```python
from build123d import *

# Parameters (mm, degrees)
EXTRUDE_1_DEPTH      = 30
EXTRUDE_1_DEPTH_BACK = 30
SKETCH_3_R           = 3.15
CUT_EXTRUDE_1_DEPTH  = 89.119294142


with BuildPart() as part:
    # Sketch 1 → Extrude 1 (new, two sides: drawn at the far end of the back side and taken through both)
    with BuildSketch(Plane.XY.offset(-EXTRUDE_1_DEPTH_BACK)):
        Polygon((-37.55, 0), (37.55, 0), (37.55, 35), (32.7, 35), (32.7, 5), (-32.7, 5), (-32.7, 35), (-37.55, 35), align=None)
    extrude(amount=EXTRUDE_1_DEPTH + EXTRUDE_1_DEPTH_BACK)

    # Sketch 3 → Cut-Extrude 1 (cut, through all)
    with BuildSketch(Plane.ZY.offset(37.55)):
        with Locations(Location((10, 27, 0), (0, 0, 270))):
            Circle(SKETCH_3_R)
        with BuildLine():
            Line((30, 5), (17.149177618, 30.590161471))
            ThreePointArc((17.149177618, 30.590161471), (14.199923108, 33.808865242), (10, 35))
            Line((10, 35), (30, 35))
            Line((30, 35), (30, 5))
        make_face()
        with BuildLine():
            ThreePointArc((-2.8, 27), (0.949033201, 17.949033201), (10, 14.2))
            ThreePointArc((10, 14.2), (12.2, 12), (10, 9.8))
            ThreePointArc((10, 9.8), (-2.162236636, 14.837763364), (-7.2, 27))
            ThreePointArc((-7.2, 27), (-5, 29.2), (-2.8, 27))
        make_face()
    extrude(amount=-CUT_EXTRUDE_1_DEPTH, mode=Mode.SUBTRACT)


solid = part.part
```
Work out the finished part from the listing and answer in its coordinate system (mm). A direction names the side the tool comes from. Round coordinates to 2 decimals unless told otherwise and drop trailing zeros. Write each loop counter-clockwise with the first axis right and the second up, starting at its lowest first coordinate (ties: lowest second). Pieces come first, ordered by that corner, then holes.
1) A cutting plane is placed at A-A on y = 21.5. Determine the outline of the cut face in (x, z), and give its area (3 significant figures).
2) Which of the six approach directions +Z, -Z, +X, -X, +Y, -Y give full straight-line access (tool end or side, diameter ignored) to faces 1 (the face through (-35, 35, -10)), 2 (the face through (-35.159, 14.705, -2.028)), 3 (the face through (0, 5, 0))?
3) A cutting plane is placed at B-B on z = -5. Determine the outline of the cut face in (x, y).
4) Determine the mould class of faces 4 (the face through (-32.7, 20, -7)), 5 (the face through (-35.2, 29.2, -5)), 6 (the face through (-1, 0, 0)), 7 (the face through (35.09, 33.78, 14.25)) for opening direction Y: pulls with the +Y half, pulls with the -Y half, needs draft (parallel to the pull), parting line crosses it, or undercut.
5) A flat-ended cylindrical pin translates along its axis: P1, Ø12, axis at x = 6, z = -16.5, coming from the +Y side. Find the tip coordinate at first contact, or state that the pin passes through.
6) A cutting plane is placed at C-C on z = 9. Determine the outline of the cut face in (x, y), and give its area (3 significant figures).
7) A cutting plane is placed at D-D on x = 29.5. Determine the outline of the cut face in (y, z), and give its area (3 significant figures).
8) Consider probe 1 along X at (y, z) = (19, -25.5); probe 2 along Z at (x, y) = (33, 27); probe 3 along Y at (x, z) = (-19, -6.5). Determine where each line is inside the solid, lowest interval first.
Entries:
1. outline: (-37.55, -30) - (-32.7, -30) - (-32.7, -6.3) - (-37.55, -6.3) - close; (-37.55, -1.56) - (-32.7, -1.56) - (-32.7, 21.71) - (-37.55, 21.71) - close; (32.7, -30) - (37.55, -30) - (37.55, -6.3) - (32.7, -6.3) - close; (32.7, -1.56) - (37.55, -1.56) - (37.55, 21.71) - (32.7, 21.71) - close
1. area: 456 mm2
2. face 1: +Z, -Z, +X, -X, +Y
2. face 2: +X, -X
2. face 3: +Z, -Z, +Y
3. outline: (-37.55, 0) - (37.55, 0) - (37.55, 18.58) - (32.7, 18.58) - (32.7, 5) - (-32.7, 5) - (-32.7, 18.58) - (-37.55, 18.58) - close; (-37.55, 29.2) - (-32.7, 29.2) - (-32.7, 35) - (-37.55, 35) - close; (32.7, 29.2) - (37.55, 29.2) - (37.55, 35) - (32.7, 35) - close
4. face 4: needs draft
4. face 5: undercut
4. face 6: pulls with the -Y half
4. face 7: pulls with the +Y half
5. P1: stops at y = 5
6. outline: (-37.55, 0) - (37.55, 0) - (37.55, 9.83) - (32.7, 9.83) - (32.7, 5) - (-32.7, 5) - (-32.7, 9.83) - (-37.55, 9.83) - close; (-37.55, 14.24) - (-32.7, 14.24) - (-32.7, 24.01) - (-37.55, 24.01) - close; (-37.55, 29.99) - (-32.7, 29.99) - (-32.7, 35) - (-37.55, 35) - close; (32.7, 14.24) - (37.55, 14.24) - (37.55, 24.01) - (32.7, 24.01) - close; (32.7, 29.99) - (37.55, 29.99) - (37.55, 35) - (32.7, 35) - close
6. area: 566 mm2
7. outline: (0, -30) - (5, -30) - (5, 30) - (0, 30) - close
7. area: 300 mm2
8. probe 1: x = -37.55 to -32.7, 32.7 to 37.55
8. probe 2: z = -30 to -7.2, -2.8 to 6.85, 13.15 to 18.95
8. probe 3: y = 0 to 5
